Source: CAD feature listing. Evaluate the final solid. Frame: model axes, mm. Face numbers are marked on the shaded views. A direction names the side the tool comes from. Coordinates: 2 decimals unless noted, no trailing zeros. Loops run counter-clockwise (first coordinate to the right, second up) from the corner with the lowest first, then second, coordinate; pieces in that order, holes last.
```python
from build123d import *

# Parameters (mm, degrees)
PAD_DEPTH = 10


with BuildPart() as part:
    # Sketch → Pad (new body)
    with BuildSketch(Plane.XZ):
        with BuildLine():
            Line((0, 0), (15, 0))
            ThreePointArc((15, 0), (18.535534, 1.464466), (20, 5))
            Line((20, 5), (20, 20))
            Line((20, 20), (25, 20))
            Line((25, 20), (25, 5))
            ThreePointArc((15, -5), (22.071068, -2.071068), (25, 5))
            Line((15, -5), (0, -5))
            Line((0, -5), (0, 0))
        make_face()
    extrude(amount=PAD_DEPTH)


solid = part.part
```
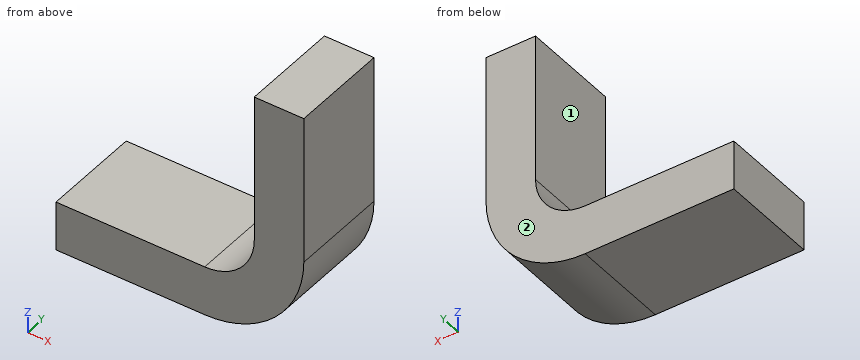
Q1. Section query A-A on y = -1.5. Return the cut outline in (x, z).
Q2. Material intervals for line 1 along Z through (x, y) = (14, -4.25); line 2 along X through (y, z) = (-4, 16); line 3 along Z through (x, y) = (21.5, -1.75), sorted ascending.
Q3. Section query B-B on z = 8.5. Return the cut outline in (x, y).
Q4. First-contact query: pin 1 Ø5 at (y, z) = (-4.5, 17) entering from -X; pin 2 Ø3 at (x, z) = (15.5, 2.5) entering from +Y. Flat tips, straight axial feed; report the tip coordinate or a pass-through.
Q5. Section query C-C on x = 12.5. Return the cut outline in (y, z), then the cut area to 3 significant figures.
Q6. Reachability of the marked faces 1 and 2 from +Z, -Z, +X, -X, +Y, -Y: full face, straight path, thin tool, end or side. Return the list, or none.
Resolved:
1. outline: (0, -5) - (15, -5) arc R10 ccw to (25, 5) - (25, 20) - (20, 20) - (20, 5) arc R5 cw to (15, 0) - (0, 0) - close
2. line 1: z = -5 to 0
2. line 2: x = 20 to 25
2. line 3: z = -2.6 to 20
3. outline: (20, -10) - (25, -10) - (25, 0) - (20, 0) - close
4. pin 1: stops at x = 20
4. pin 2: passes through
5. outline: (-10, -5) - (0, -5) - (0, 0) - (-10, 0) - close
5. area: 50.0 mm2
6. face 1: +Z, -X, +Y, -Y
6. face 2: +Z, -Z, +X, -X, +Y
